The listing builds one solid part. Answer for the finished solid, in the listing's coordinates (mm). Face numbers are marked on the shaded views. A direction names the side the tool comes from. Round coordinates to 2 decimals unless told otherwise and drop trailing zeros. Order: outer loops, then holes, each group sorted by start corner. A loop starts at its lowest first (then second) coordinate and runs counter-clockwise, first axis right, second up. Notation, with made-up numbers: (36, -37.75) - (61, -37.75) arc R31 ccw to (61, -9.75) - close; hole circle Ø11 at (-26, 34). An arc over 180 degrees is marked (long way). Use CSV: the item, a comma, the result in double quotes. Start each with the question number.
Item 1: Straight lines are drawn through the part: line 1 along X through (y, z) = (0.75, 10.5); line 2 along Y through (x, z) = (2, 1.25); line 3 along Z through (x, y) = (-2.75, -2.25). For each, find the intervals that lie inside material, in ascending order. Write a range as [from, to].
Item 2: Find section B-B, the plane z = 9.25. Give the vertices of the cut face in (x, y), plus the area to 3 significant figures.
Item 3: Flat-ended cylindrical pins translate along their axes: P1, Ø2, axis at x = 2, z = 5.5, coming from the -Y side; P2, Ø1, axis at y = -1, z = 10, coming from the +X side; P3, Ø1.3, axis at x = -0.5, z = 11, coming from the +Y side. Find the tip coordinate at first contact, or state that the pin passes through.
Item 4: Find section D-D, the plane z = 2.25. Give the vertices of the cut face in (x, y).
Item 5: Find section C-C, the plane y = 0. Give the vertices of the cut face in (x, z), plus the area to 3 significant figures.
Item 6: For the marked faces 4 and 5, determine the directions among +Z, -Z, +X, -X, +Y, -Y from which every point of the face is accessible in a straight line to the end or side of a thin tool.
Item 7: Find section A-A, the plane x = 0. Give the vertices of the cut face in (y, z).
Item 8: Determine the mould class of the marked faces 1, 2 and 3 for opening direction Y: +Y half, -Y half, draft (parallel to the pull), parting line (faces both ways), or undercut.
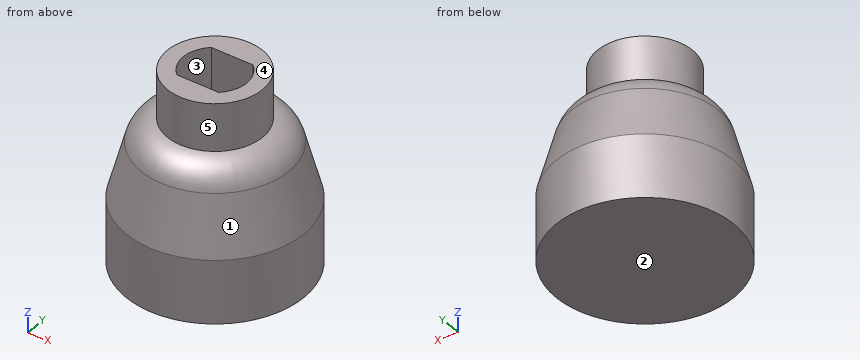
```python
from build123d import *

# Parameters (mm, degrees)
SKETCH1_R           = 5.6
BOSS_EXTRUDE1_DEPTH = 9
SKETCH2_R           = 3
BOSS_EXTRUDE2_DEPTH = 3
CHAMFER1_SIZE       = 5
CHAMFER1_SIZE2      = 1.339745962


with BuildPart() as part:
    # Sketch1 → Boss-Extrude1 (new body)
    with BuildSketch(Plane.XY):
        Circle(SKETCH1_R)
    extrude(amount=BOSS_EXTRUDE1_DEPTH)

    # Sketch2 → Boss-Extrude2 (add)
    with BuildSketch(Plane.XY.offset(9)):
        Circle(SKETCH2_R)
        with BuildLine():
            Line((-1.322875656, -1.5), (1.322875656, -1.5))
            ThreePointArc((1.322875656, -1.5), (2, 0), (1.322875656, 1.5))
            Line((1.322875656, 1.5), (-1.322875656, 1.5))
            ThreePointArc((-1.322875656, 1.5), (-2, 0), (-1.322875656, -1.5))
        make_face(mode=Mode.SUBTRACT)
    extrude(amount=BOSS_EXTRUDE2_DEPTH)

    # Chamfer1
    chamfer1_edges = [part.edges().sort_by_distance(p)[0] for p in [
        (-5.6, 0, 9),
    ]]
    chamfer1_side = [part.faces().sort_by_distance(p)[0] for p in [
        (-5.6, 0, 4.5),
    ]]
    chamfer(chamfer1_edges, length=CHAMFER1_SIZE, length2=CHAMFER1_SIZE2, reference=chamfer1_side[0])

    # Fillet1: read off the stored shape, not the designer's step
    # Fillet1 outline → Fillet1 (revolve, cut)
    with BuildSketch(Plane.XZ):
        with BuildLine():
            Line((4.652186603, 7.537287752), (4.652186603, 9))
            Line((4.652186603, 9), (3, 9))
            ThreePointArc((3, 9), (4.04607373, 8.517119759), (4.652186603, 7.537287752))
        make_face()
    revolve(axis=Axis((0, 0, 0), (0, 0, 1)), mode=Mode.SUBTRACT)


solid = part.part
```
Worked out:
1,line 1,"x = [-2.9, -1.85], [1.85, 2.9]"
1,line 2,"y = [-5.23, 5.23]"
1,line 3,"z = [0, 8.84]"
2,outline,"circle Ø6 at (0, 0); hole (-1.32, -1.5) - (1.32, -1.5) arc R2 ccw to (1.32, 1.5) - (-1.32, 1.5) arc R2 ccw to start"
2,area,"17.5 mm²"
3,P1,"stops at y = -5.23"
3,P2,"stops at x = 2.96"
3,P3,"stops at y = 3"
4,outline,"circle Ø11.2 at (0, 0)"
5,outline,"(-5.6, 0) - (5.6, 0) - (5.6, 4) - (4.65, 7.54) arc R2 ccw to (3, 9) - (3, 12) - (2, 12) - (2, 9) - (-2, 9) - (-2, 12) - (-3, 12) - (-3, 9) arc R2 ccw to (-4.65, 7.54) - (-5.6, 4) - close"
5,area,"99.3 mm²"
6,face 4,"+Z, +X, -X, +Y, -Y"
6,face 5,"+Z"
7,outline,"(-5.6, 0) - (5.6, 0) - (5.6, 4) - (4.65, 7.54) arc R2 ccw to (3, 9) - (3, 12) - (1.5, 12) - (1.5, 9) - (-1.5, 9) - (-1.5, 12) - (-3, 12) - (-3, 9) arc R2 ccw to (-4.65, 7.54) - (-5.6, 4) - close"
8,face 1,"parting line"
8,face 2,"draft"
8,face 3,"undercut"
